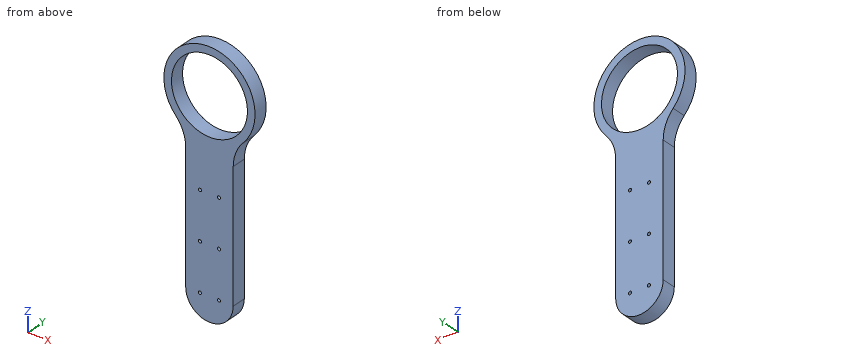
```python
from build123d import *

# Parameters (mm, degrees)
SKETCH1_R           = 39.9935
BOSS_EXTRUDE1_DEPTH = 15
SKETCH2_R           = 1.65
CUT_EXTRUDE1_DEPTH  = 15


with BuildPart() as part:
    # Sketch1 → Boss-Extrude1 (new body)
    with BuildSketch(Plane(origin=(0, 0, 0), x_dir=(1, 0, 0), z_dir=(0, 1, 0))):
        with BuildLine():
            Line((25, 59.311516944), (25, 195))
            ThreePointArc((25, 195), (0, 220), (-25, 195))
            Line((-25, 195), (-25, 59.311516944))
            ThreePointArc((-25, 59.311516944), (-27.704521174, 44.853050249), (-35.452362959, 32.349745021))
            ThreePointArc((-35.452362959, 32.349745021), (0, -47.9935), (35.452362959, 32.349745021))
            ThreePointArc((35.452362959, 32.349745021), (27.704521174, 44.853050249), (25, 59.311516944))
        make_face()
        with Locations(Location((0, 0, 0), (0, 0, 270))):
            Circle(SKETCH1_R, mode=Mode.SUBTRACT)
    extrude(amount=BOSS_EXTRUDE1_DEPTH)

    # Sketch2 → Cut-Extrude1 (cut)
    with BuildSketch(Plane.XZ):
        with Locations(Location((10, -95, 0), (0, 0, 270))):
            Circle(SKETCH2_R)
        with Locations(Location((-10, -95, 0), (0, 0, 270))):
            Circle(SKETCH2_R)
        with Locations(Location((10, -145, 0), (0, 0, 270))):
            Circle(SKETCH2_R)
        with Locations(Location((-10, -145, 0), (0, 0, 270))):
            Circle(SKETCH2_R)
        with Locations(Location((10, -195, 0), (0, 0, 270))):
            Circle(SKETCH2_R)
        with Locations(Location((-10, -195, 0), (0, 0, 270))):
            Circle(SKETCH2_R)
    extrude(amount=-CUT_EXTRUDE1_DEPTH, mode=Mode.SUBTRACT)


solid = part.part
```
Could you check a few things on this model? Use its own coordinates, in mm. Coordinates: 2 decimals unless noted, no trailing zeros. Order: outer loops, then holes, each group sorted by start corner. A loop starts at its lowest first (then second) coordinate and runs counter-clockwise, first axis right, second up. Notation, with made-up numbers: M -31,12.25 L 27,12.25 A16 cw 27,22.25 Z; hole C 55.5,-35.5 d3. An arc over 180 degrees is marked long. Use a Markdown table: item, result. Add a question column.
Q1. I'm going to push flat-ended pins straight in: pin 1 (2 mm diameter, centred on x = -10, z = -195, fed in from -Y); pin 2 (4 mm diameter, centred on y = 5, z = -102, fed in from +X); pin 3 (8 mm diameter, centred on y = 2, z = -106.5, fed in from -X); pin 4 (6 mm diameter, centred on x = -36, y = 10.5, fed in from +Z). Where does each tip first touch, or does it pass through?
Q2. I want a section at C-C on x = 22.5. List the corners of the cut face in (y, z) for me, then the cut area to 3 significant figures.
Q3. I want a section at D-D on z = -85. List the corners of the cut face in (x, y) for me.
Q4. I want a section at A-A on z = 0. List the corners of the cut face in (x, y) for me.
Q5. I want a section at B-B on y = 2.75. List the corners of the cut face in (x, z) for me, then the cut area to 3 significant figures.
Q6. If I drill on L1, parallel to X at y = 11, z = -195; L2, parallel to X at y = 2.5, z = 2; L3, parallel to Z at x = -0.5, y = 13 (3 decimals), over which ranges is the centre line in solid material (lowest first)?
Checked values:
| question | item | result |
|---|---|---|
| 1 | pin 1 | through |
| 1 | pin 2 | x = 25 |
| 1 | pin 3 | x = -25 |
| 1 | pin 4 | z = 34.85 |
| 2 | outline | M 0,-205.9 L 15,-205.9 L 15,-33.06 L 0,-33.06 Z; M 0,33.06 L 15,33.06 L 15,42.39 L 0,42.39 Z |
| 2 | area | 2,730 mm² |
| 3 | outline | M -25,0 L 25,0 L 25,15 L -25,15 Z |
| 4 | outline | M -47.99,0 L -39.99,0 L -39.99,15 L -47.99,15 Z; M 39.99,0 L 47.99,0 L 47.99,15 L 39.99,15 Z |
| 5 | outline | M -35.45,-32.35 A40 cw -25,-59.31 L -25,-195 A25 ccw 25,-195 L 25,-59.31 A40 cw 35.45,-32.35 A47.99 ccw long Z; hole C 0,0 d79.99; hole C -10,-195 d3.3; hole C -10,-145 d3.3; hole C -10,-95 d3.3; hole C 10,-195 d3.3; hole C 10,-145 d3.3; hole C 10,-95 d3.3 |
| 5 | area | 10,700 mm² |
| 6 | L1 | -25 to -11.65, -8.35 to 8.35, 11.65 to 25 |
| 6 | L2 | -47.95 to -39.94, 39.94 to 47.95 |
| 6 | L3 | -219.995 to -39.99, 39.99 to 47.991 |
